```python
from build123d import *

# Parameters (mm, degrees)
F0_W     = 342.9
F0_H     = 723.9
F1_DEPTH = 12.7
F2_W     = 266.7
F2_H     = 647.7
F2_W_2   = 241.3
F2_H_2   = 622.3
F3_DEPTH = 6.35
F4_R     = 5.08


with BuildPart() as f1:
    # F0 (on Front) → F1 (new body)
    with BuildSketch(Plane.XZ):
        with Locations((-45.644873, -8.329587)):
            Rectangle(F0_W, F0_H)
    extrude(amount=F1_DEPTH)

    # F2 (on face) → F3 (cut)
    with BuildSketch(Plane.XZ.offset(12.7)):
        with Locations((-45.644873, -8.329587)):
            Rectangle(F2_W, F2_H)
        with Locations((-45.644873, -8.329587)):
            Rectangle(F2_W_2, F2_H_2, mode=Mode.SUBTRACT)
    extrude(amount=-F3_DEPTH, mode=Mode.SUBTRACT)

    # F4
    f4_edges = [f1.edges().sort_by_distance(p)[0] for p in [
        (-217.094873, -12.7, -8.329587),
        (-45.644873, -12.7, 353.620413),
        (125.805127, -12.7, -8.329587),
        (87.705127, -12.7, -8.329587),
        (-45.644873, -12.7, 315.520413),
        (-178.994873, -12.7, -8.329587),
        (-166.294873, -12.7, -8.329587),
        (-45.644873, -12.7, 302.820413),
        (75.005127, -12.7, -8.329587),
        (-45.644873, -12.7, -319.479587),
        (-45.644873, -12.7, -332.179587),
    ]]
    fillet(f4_edges, radius=F4_R)


solid = f1.part
```
Design review of the part built by this model. Coordinates are the model's own, in mm. Give positions to 0.01 mm unless a question says otherwise; leave off trailing zeros. Loops run counter-clockwise (first coordinate to the right, second up) from the corner with the lowest first, then second, coordinate; pieces in that order, holes last. Notation, with made-up numbers: M 9,-17 L 35,-17 A33 cw 35,16 Z; hole C -4,47 d1. An arc over 180 degrees is marked long. Return JSON: item names as keys, results as strings. Group by question number.
Item 1: For probe 1 along X at (y, z) = (-8, 215.5); probe 2 along Z at (x, y) = (-150.5, -8); probe 3 along Z at (x, y) = (22.5, -8.5), list the stretches that pass through material, from the lowest coordinate up.
Item 2: We need section C-C (x = -57). Give the boundary of the cut face in (y, z).
Item 3: We need section B-B (z = -109.5). Give the boundary of the cut face in (x, y), and give its area (3 significant figures).
Item 4: We need section A-A (y = -10.5). Give the boundary of the cut face in (x, z).
Item 5: Insertion check: pin 1 Ø4 at (x, y) = (-111.5, -10.5) entering from +Z. The pin has a flat end and moves straight along its axis. Give the tip position at first contact, or say it passes through.
Item 6: Mouldability with a two-part tool opening along X and no side actions: class faces 1 (the flat face through (-194, -12.7, 17)), 2 (the flat face through (82, -6.35, 89)) as released by +X, released by -X, zero draft, split by the parting line, or undercut.
Output:
{
 "1": {"probe 1": "x = -217.08 to -179.01, -166.28 to 74.99, 87.72 to 125.79", "probe 2": "z = -370.28 to -332.19, -319.47 to 302.81, 315.53 to 353.61", "probe 3": "z = -370.28 to -332.26, -319.4 to 302.74, 315.6 to 353.54"},
 "2": {"outline": "M -12.7,-370.28 L 0,-370.28 L 0,353.62 L -7.62,353.62 A5.08 ccw -12.7,348.54 L -12.7,320.6 A5.08 ccw -7.62,315.52 L -6.35,315.52 L -6.35,302.82 L -7.62,302.82 A5.08 ccw -12.7,297.74 L -12.7,-314.4 A5.08 ccw -7.62,-319.48 L -6.35,-319.48 L -6.35,-332.18 L -7.62,-332.18 A5.08 ccw -12.7,-337.26 Z"},
 "3": {"outline": "M -217.09,-7.62 A5.08 ccw -212.01,-12.7 L -184.07,-12.7 A5.08 ccw -178.99,-7.62 L -178.99,-6.35 L -166.29,-6.35 L -166.29,-7.62 A5.08 ccw -161.21,-12.7 L 69.93,-12.7 A5.08 ccw 75.01,-7.62 L 75.01,-6.35 L 87.71,-6.35 L 87.71,-7.62 A5.08 ccw 92.79,-12.7 L 120.73,-12.7 A5.08 ccw 125.81,-7.62 L 125.81,0 L -217.09,0 Z", "area": "4,160 mm^2"},
 "4": {"outline": "M -216.2,-370.28 L 124.91,-370.28 L 124.91,352.73 L -216.2,352.73 Z; M -165.4,-318.58 L 74.11,-318.58 L 74.11,301.93 L -165.4,301.93 Z; hole M -179.89,-333.07 L 88.6,-333.07 L 88.6,316.42 L -179.89,316.42 Z"},
 "5": {"pin 1": "stops at z = 353.54"},
 "6": {"face 1": "zero draft", "face 2": "undercut"}
}
